For this review, use the dimensioned drawing (mm, ordinates from the lowest corner) and the shaded views. A direction names the side the tool comes from. Coordinates: 2 decimals unless noted, no trailing zeros. Write each loop counter-clockwise with the first axis right and the second up, starting at its lowest first coordinate (ties: lowest second). Pieces come first, ordered by that corner, then holes. Notation, with made-up numbers: (42.5, 24) - (92.5, 24) arc R19 ccw to (92.5, 50) - close; hole circle Ø3 at (67.5, 88). An arc over 180 degrees is marked (long way). Answer as a JSON object with one key per item and string values.
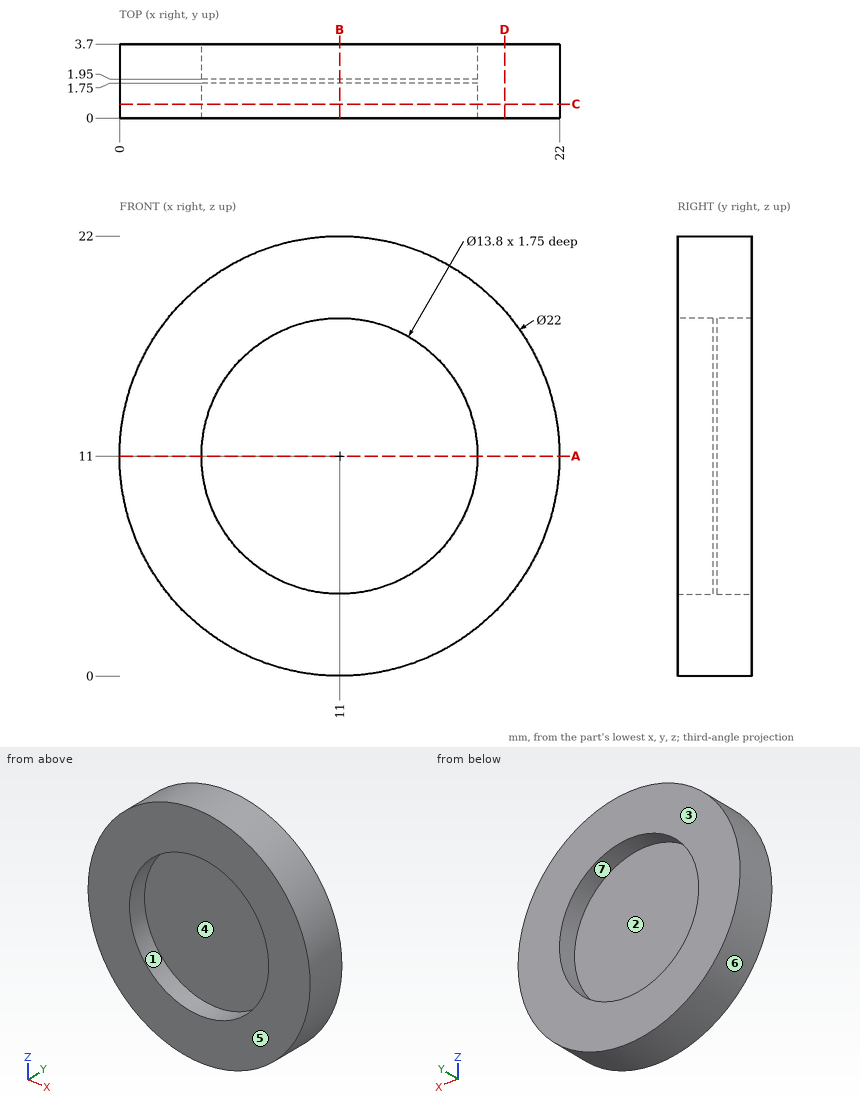
(1) To check wall thickness, follow line 1 (X direction, y = 3.25, z = 11); line 2 (Z direction, x = 11.5, y = 3.4); line 3 (X direction, y = 0.7, z = 12). State the ranges of each line that lie inside material, in increasing order. Write a range as from..to.
Solved:
{"line 1": "x = 0..4.1, 17.9..22", "line 2": "z = 0.01..4.12, 17.88..21.99", "line 3": "x = 0.05..4.17, 17.83..21.95"}
(2) The part is to be moulded in two halves that separate along X. For the marked faces 4, 5, 6 and 7, say which applies: pulls with the +X half, pulls with the -X half, needs draft (parallel to the pull), parting line crosses it, or undercut.
Solved:
{"face 4": "undercut", "face 5": "needs draft", "face 6": "parting line crosses it", "face 7": "undercut"}
(3) For pin 1 (2 mm diameter, centred on y = 3, z = 19, fed in from +X); pin 2 (3 mm diameter, centred on x = 7, z = 10, fed in from +Y); pin 3 (2 mm diameter, centred on x = 14.5, y = 3, fed in from +Z), all flat-tipped, find the tip position at first contact; note any pin that passes through.
Solved:
{"pin 1": "stops at x = 19.49", "pin 2": "stops at y = 1.95", "pin 3": "stops at z = 21.71"}
(4) Take a section at B-B, the plane x = 11. Write out the cut boundary in (y, z), and give its area (3 significant figures).
Solved:
{"outline": "(0, 0) - (3.7, 0) - (3.7, 4.1) - (1.95, 4.1) - (1.95, 17.9) - (3.7, 17.9) - (3.7, 22) - (0, 22) - (0, 17.9) - (1.75, 17.9) - (1.75, 4.1) - (0, 4.1) - close", "area": "33.1 mm^2"}
(5) Take a section at D-D, the plane x = 19.25. Write out the cut boundary in (y, z), and give its area (3 significant figures).
Solved:
{"outline": "(0, 3.72) - (3.7, 3.72) - (3.7, 18.28) - (0, 18.28) - close", "area": "53.8 mm^2"}
(6) Tool access review of the marked faces 1, 2 and 3: name each direction out of +Z, -Z, +X, -X, +Y, -Y from which nothing blocks a thin tool from reaching the whole face with its end or side.
Solved:
{"face 1": "-Y", "face 2": "+Y", "face 3": "+Z, -Z, +X, -X, +Y"}
(7) Take a section at A-A, the plane z = 11. Write out the cut boundary in (x, y).
Solved:
{"outline": "(0, 0) - (4.1, 0) - (4.1, 1.75) - (17.9, 1.75) - (17.9, 0) - (22, 0) - (22, 3.7) - (17.9, 3.7) - (17.9, 1.95) - (4.1, 1.95) - (4.1, 3.7) - (0, 3.7) - close"}
(8) Take a section at C-C, the plane y = 0.7. Write out the cut boundary in (x, z).
Solved:
{"outline": "circle Ø22 at (11, 11); hole circle Ø13.8 at (11, 11)"}
